from build123d import *

# Parameters (mm, degrees)
F0_R     = 3
F1_DEPTH = 10
F2_SIZE  = 1.5
F3_SIZE  = 1


with BuildPart() as f1:
    # F0 (on Right) → F1 (new body)
    with BuildSketch(Plane.YZ):
        with Locations((0, 3)):
            Circle(F0_R)
    extrude(amount=F1_DEPTH)

    # F2
    f2_edges = [f1.edges().sort_by_distance(p)[0] for p in [
        (10, -3, 3),
    ]]
    chamfer(f2_edges, length=F2_SIZE)

    # F3
    f3_edges = [f1.edges().sort_by_distance(p)[0] for p in [
        (0, -3, 3),
    ]]
    chamfer(f3_edges, length=F3_SIZE)


solid = f1.part
Input: part model. Units: mm. Frame: model coordinates. Give positions to 0.01 mm unless a question says otherwise; leave off trailing zeros. Order: outer loops, then holes, each group sorted by start corner. A loop starts at its lowest first (then second) coordinate and runs counter-clockwise, first axis right, second up. Notation, with made-up numbers: (12, 43.5) - (48, 43.5) arc R21 cw to (48, 47.5) - close; hole circle Ø4 at (-27.75, 23). An arc over 180 degrees is marked (long way). Answer as a JSON object with one key per item and string values. Group by question number.
Q1. Cut plane B-B, the plane y = 0. Output: boundary loops of the cut face in (x, z).
Q2. Line query: probe 1 along Z at (x, y) = (7, 0.7); probe 2 along Y at (x, z) = (5, 5.1); probe 3 along X at (y, z) = (0.85, 1.15). Output: solid intervals per line, ascending.
Q3. Cut plane D-D, the plane x = 7.25. Output: boundary loops of the cut face in (y, z), then the cut area to 3 significant figures.
Q4. First-contact query: pin 1 Ø3 at (y, z) = (0.5, 4) entering from -X. Flat tip, straight axial feed; report the tip coordinate or a pass-through.
Q5. Cut plane A-A, the plane z = 3. Output: boundary loops of the cut face in (x, y), then the cut area to 4 significant figures.
Q6. Cut plane C-C, the plane x = 9.25. Output: boundary loops of the cut face in (y, z), then the cut area to 3 significant figures.
Results:
{
 "1": {"outline": "(0, 1) - (1, 0) - (8.5, 0) - (10, 1.5) - (10, 4.5) - (8.5, 6) - (1, 6) - (0, 5) - close"},
 "2": {"probe 1": "0.08 to 5.92", "probe 2": "-2.14 to 2.14", "probe 3": "0.04 to 9.46"},
 "3": {"outline": "circle Ø6 at (0, 3)", "area": "28.3 mm^2"},
 "4": {"pin 1": "x = 0"},
 "5": {"outline": "(0, -2) - (1, -3) - (8.5, -3) - (10, -1.5) - (10, 1.5) - (8.5, 3) - (1, 3) - (0, 2) - close", "area": "56.75 mm^2"},
 "6": {"outline": "circle Ø4.5 at (0, 3)", "area": "15.9 mm^2"}
}
